from build123d import *

# Parameters (mm, degrees)
KREISMUSTER1_COUNT = 4


with BuildPart() as part:
    # Skizze1 → Rotation1 (revolve)
    with BuildSketch(Plane.XY):
        Polygon((0, 37.5), (0, 16), (2, 16), (2, 21.5), (4, 21.5), (4, 23.5), (2, 23.5), (2, 37.5), align=None)
    revolve(axis=Axis((-7.743389997, 0, 0), (1, 0, 0)))

    # Skizze7 → Ø5.2 (5.2) Durchmesser Bohrung1 (revolve, cut)
    with BuildSketch(Plane.ZX.offset(32.5)):
        Polygon((0, 0), (0, 31.562237609), (2.6, 30), (2.6, 0), align=None)
    f_5_2_5_2_durchmesser_bohrung1 = revolve(axis=Axis((-6.35, 32.5, 0), (1, 0, 0)), mode=Mode.SUBTRACT)

    # Kreismuster1: Ø5.2 (5.2) Durchmesser Bohrung1 ×4 about axis
    kreismuster1_axis = Axis((0, 0, 0), (1, 0, 0))
    for i in range(1, KREISMUSTER1_COUNT):
        add(f_5_2_5_2_durchmesser_bohrung1.rotate(kreismuster1_axis, i * 360 / KREISMUSTER1_COUNT), mode=Mode.SUBTRACT)


solid = part.part
The listing builds one solid part. Answer for the finished solid, in the listing's coordinates (mm). A direction names the side the tool comes from. Round coordinates to 2 decimals unless told otherwise and drop trailing zeros. Write each loop counter-clockwise with the first axis right and the second up, starting at its lowest first coordinate (ties: lowest second). Pieces come first, ordered by that corner, then holes. Notation, with made-up numbers: M 45,78 L 51,78 A30 ccw 51,106 Z; hole C 0,88.25 d4. An arc over 180 degrees is marked long. Write each question's results on one line, items separated by ' | '. Start each with the question number.
Item 1: Find section A-A on y = 0. Write down the section's boundary in (x, z).
Item 2: Straight lines are drawn through the part: probe 1 along Z at (x, y) = (1.2, 0); probe 2 along Y at (x, z) = (3.2, -0.5); probe 3 along X at (y, z) = (25, 3). For each, find the intervals that lie inside material, in ascending order.
Item 3: Find section C-C on x = 0.8. Write down the section's boundary in (y, z), and give its area (3 significant figures).
Item 4: Given pin 1 Ø4 at (y, z) = (-11, -26) entering from +X; pin 2 Ø1.5 at (x, z) = (2.5, 18) entering from +Y, each flat-ended and moving along its own axis, determine where each tip first touches the part or whether it passes through.
Item 5: Which of the six approach directions +Z, -Z, +X, -X, +Y, -Y give full straight-line access (tool end or side, diameter ignored) to faces 1 (the cylindrical face through (3.014, -2.799, 21.317)), 2 (the cylindrical face through (0.986, -29.922, 0.338))?
Item 6: Find section D-D on y = -32.5. Write down the section's boundary in (x, z).
Item 7: The mould has two halves that part along Y. Classify faces 3 (the flat face through (4, -10.33, -19.04)), 4 (the cylindrical face through (0.986, -0.338, -29.922)), 5 (the cylindrical face through (3, 22.4, 7.1)): +Y half, -Y half, draft (parallel to the pull), parting line (faces both ways), or undercut.
Answer block:
1) outline: M 0,-37.5 L 2,-37.5 L 2,-35.1 L 0,-35.1 Z; M 0,-29.9 L 2,-29.9 L 2,-23.5 L 4,-23.5 L 4,-21.5 L 2,-21.5 L 2,-16 L 0,-16 Z; M 0,16 L 2,16 L 2,21.5 L 4,21.5 L 4,23.5 L 2,23.5 L 2,29.9 L 0,29.9 Z; M 0,35.1 L 2,35.1 L 2,37.5 L 0,37.5 Z
2) probe 1: z = -37.5 to -35.1, -29.9 to -16, 16 to 29.9, 35.1 to 37.5 | probe 2: y = -23.49 to -21.49, 21.49 to 23.49 | probe 3: x = 0 to 2
3) outline: C 0,0 d75; hole C -32.5,0 d5.2; hole C 0,0 d32; hole C 0,-32.5 d5.2; hole C 0,32.5 d5.2; hole C 32.5,0 d5.2 | area: 3,530 mm²
4) pin 1: stops at x = 2 | pin 2: stops at y = 33.2
5) face 1: +X | face 2: +X, -X
6) outline: M 0,-18.71 L 2,-18.71 L 2,-2.6 L 0,-2.6 Z; M 0,2.6 L 2,2.6 L 2,18.71 L 0,18.71 Z
7) face 3: draft | face 4: undercut | face 5: parting line
